Can you work these out from the model? Positions are in its coordinate system, mm. Face numbers are marked on the shaded views. Coordinates: 2 decimals unless noted, no trailing zeros. Order: outer loops, then holes, each group sorted by start corner. A loop starts at its lowest first (then second) coordinate and runs counter-clockwise, first axis right, second up. Notation, with made-up numbers: (-14.5, 43.25) -> (-6.5, 43.25) arc R29 ccw to (-6.5, 68.25) -> close; hole circle Ø8 at (64, 51.25). An arc over 180 degrees is marked (long way). Use a Markdown table: item, result. Add a question column.
1. Suppose I cut it at A-A, the plane x = 0. State how many separate pieces and enclosed holes the cut face has, then the cut area to 3 significant figures.
2. Suppose I cut it at C-C, the plane x = 152.5. List the corners of the cut face in (y, z) for me.
3. We'd pull the mould along Y, two halves only. Please class the marked faces 1, 2 and 3: pulls with the +Y half, pulls with the -Y half, needs draft (parallel to the pull), parting line crosses it, or undercut.
4. If I drill on line 1 along Y through (x, z) = (0, -20); line 2 along X through (y, z) = (0, -19); line 3 along X through (y, z) = (-5, -22.25), over which ranges is the centre line in solid material (lowest first)? Write a range as from..to.
5. For pin 1 Ø9.5 at (x, y) = (74, 2.5) entering from +Z; pin 2 Ø6 at (y, z) = (28, -5.5) entering from +X; pin 3 Ø12 at (x, y) = (-100, 16) entering from +Z, each with a flat end and sliding along its axis, tell me the tip position at first contact or that it passes through.
```python
from build123d import *

# Parameters (mm, degrees)
F1_W     = 254
F1_H     = 127
F1_R     = 50.8
F2_DEPTH = 25.4
F5_DEPTH = 127.001
F3_W     = 22.938862443
F3_H     = 126.9670481086
F3_W_2   = 76.2
F3_H_2   = 126.8606091142
F7_DEPTH = 10.414
F7_TAPER = -3
F6_R     = 10.16
F8_DEPTH = 76.2


with BuildPart() as f2:
    # F1 (on face) → F2 (new body)
    with BuildSketch(Plane.XY):
        Rectangle(F1_W, F1_H)
        Circle(F1_R, mode=Mode.SUBTRACT)
    extrude(amount=-F2_DEPTH)

    # F4 (on face) → F5 (cut, through all)
    with BuildSketch(Plane.XZ.offset(63.5)):
        Polygon((86.36, 0), (66.04, 0), (60.174121265, -10.16), (92.225878735, -10.16), align=None)
    extrude(amount=-F5_DEPTH, mode=Mode.SUBTRACT)

    # F3 (on face) → F7 (cut)
    with BuildSketch(Plane.XY):
        with Locations((-100.2905687785, 0.0164759457)):
            Rectangle(F3_W, F3_H)
        with Locations((0, 0.0696954429)):
            Rectangle(F3_W_2, F3_H_2)
    extrude(amount=-F7_DEPTH, taper=F7_TAPER, mode=Mode.SUBTRACT)

    # F6 (on face) → F8 (join)
    with BuildSketch(Plane.YZ.offset(127)):
        with Locations((0, -12.7)):
            Circle(F6_R)
    extrude(amount=F8_DEPTH)


solid = f2.part
```
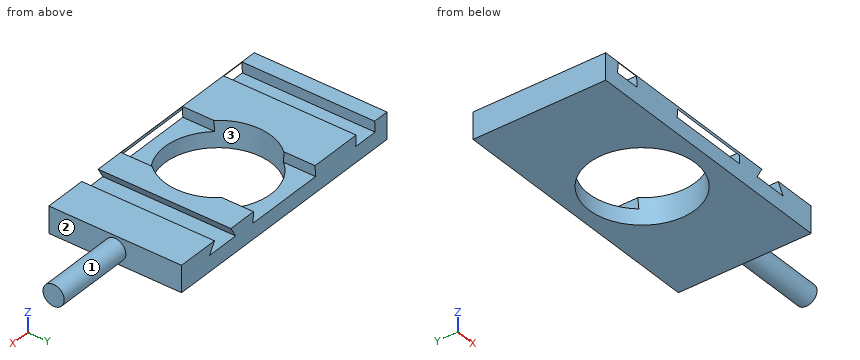
Worked out:
| question | item | result |
|---|---|---|
| 1 | separate pieces | 3 |
| 1 | enclosed holes | 0 |
| 1 | area | 381 mm² |
| 2 | outline | circle Ø20.32 at (0, -12.7) |
| 3 | face 1 | parting line crosses it |
| 3 | face 2 | needs draft |
| 3 | face 3 | undercut |
| 4 | line 1 | y = -63.5..-50.8, 50.8..63.5 |
| 4 | line 2 | x = -127..-50.8, 50.8..203.2 |
| 4 | line 3 | x = -127..-50.55, 50.55..127 |
| 5 | pin 1 | stops at z = -10.16 |
| 5 | pin 2 | stops at x = 127 |
| 5 | pin 3 | stops at z = -10.41 |
